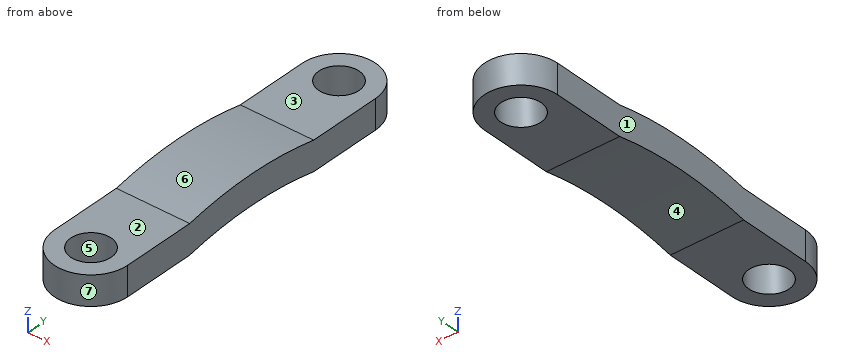
```python
from build123d import *

# Parameters (mm, degrees)
F1_DEPTH = 4
F2_D     = 5.5
F2_DEPTH = 7
F2_TIP   = 1.6523667023
F3_W     = 5
F3_H     = 4
F4_DEPTH = 5
F6_DEPTH = 4
F7_D     = 5.5
F7_DEPTH = 7
F7_TIP   = 1.6523667023


with BuildPart() as f1:
    # F0 (on Top) → F1 (new body)
    with BuildSketch(Plane.XY):
        with BuildLine():
            Line((-5, 5), (-5, 0))
            ThreePointArc((-5, 0), (0, -5), (5, 0))
            Line((5, 0), (5, 5))
            Line((5, 5), (-5, 5))
        make_face()
    extrude(amount=F1_DEPTH)

    # F2
    with Locations(Plane(origin=(0, 0, 0), x_dir=(1, 0, 0), z_dir=(0, 0, -1))):
        with Locations((0, 0)):
            Hole(F2_D / 2, depth=F2_DEPTH)
            with Locations((0, 0, -(F2_DEPTH + F2_TIP / 2))):  # 118° drill point
                Cone(0, F2_D / 2, F2_TIP, mode=Mode.SUBTRACT)

    # F3 (on Right) → F4 (join, symmetric)
    with BuildSketch(Plane.YZ):
        with Locations((7.5, 2)):
            Rectangle(F3_W, F3_H)
        with BuildLine():
            Line((10, 4), (10, 0))
            ThreePointArc((10, 0), (14.9745518997, 0.7570127946), (20, 1.0102051443))
            Line((20, 1.0102051443), (20, 5.0102051443))
            ThreePointArc((20, 5.0102051443), (14.9745518997, 4.7570127946), (10, 4))
        make_face()
        with BuildLine():
            Line((20, 5.0102051443), (20, 1.0102051443))
            ThreePointArc((20, 1.0102051443), (25.0254481003, 0.7570127946), (30, 0))
            Line((30, 0), (30, 4))
            ThreePointArc((30, 4), (25.0254481003, 4.7570127946), (20, 5.0102051443))
        make_face()
        with Locations((32.5, 2)):
            Rectangle(F3_W, F3_H)
    extrude(amount=F4_DEPTH, both=True)

    # F5 (on Top) → F6 (join)
    with BuildSketch(Plane.XY):
        with BuildLine():
            Line((5, 35), (5, 40))
            ThreePointArc((5, 40), (0, 45), (-5, 40))
            Line((-5, 40), (-5, 35))
            Line((-5, 35), (5, 35))
        make_face()
    extrude(amount=F6_DEPTH)

    # F7
    with Locations(Plane(origin=(0, 0, 0), x_dir=(1, 0, 0), z_dir=(0, 0, -1))):
        with Locations((0, -40)):
            Hole(F7_D / 2, depth=F7_DEPTH)
            with Locations((0, 0, -(F7_DEPTH + F7_TIP / 2))):  # 118° drill point
                Cone(0, F7_D / 2, F7_TIP, mode=Mode.SUBTRACT)


solid = f1.part
```
Model file for the job. Use its own axes, mm. Face numbers are marked on the shaded views. A direction names the side the tool comes from. Round coordinates to 2 decimals unless told otherwise and drop trailing zeros. Order: outer loops, then holes, each group sorted by start corner. A loop starts at its lowest first (then second) coordinate and runs counter-clockwise, first axis right, second up. Notation, with made-up numbers: (-39.75, 25) -> (-24.75, 25) arc R16 cw to (-24.75, 47) -> close; hole circle Ø6 at (69, 78.5). An arc over 180 degrees is marked (long way). Use one line per item in the form item = value.
Item 1: Cut at B-B, the plane x = 0. Write the cut outline in (y, z), and give its area (3 significant figures).
Returned:
outline = (-5, 0) -> (-2.75, 0) -> (-2.75, 4) -> (-5, 4) -> close; (2.75, 0) -> (10, 0) arc R50 cw to (30, 0) -> (37.25, 0) -> (37.25, 4) -> (30, 4) arc R50 ccw to (10, 4) -> (2.75, 4) -> close; (42.75, 0) -> (45, 0) -> (45, 4) -> (42.75, 4) -> close
area = 156 mm^2
Item 2: Cut at A-A, the plane z = 0.45. Write the cut outline in (x, y).
Returned:
outline = (-5, 0) arc R5 ccw to (5, 0) -> (5, 12.54) -> (-5, 12.54) -> close; (-5, 27.46) -> (5, 27.46) -> (5, 40) arc R5 ccw to (-5, 40) -> close; hole circle Ø5.5 at (0, 0); hole circle Ø5.5 at (0, 40)
Item 3: Pull direction Y, two halves, no side cores. Call the marked faces 4, 5, 6 and 7: released by +Y, released by -Y, zero draft, split by the parting line, or undercut.
Returned:
face_4 = undercut
face_5 = undercut
face_6 = split by the parting line
face_7 = released by -Y
Item 4: Flat gauge pins, fed straight in: pin 1 Ø3 at (x, y) = (-0.5, 6) entering from +Z; pin 2 Ø1.5 at (x, z) = (4, 2.5) entering from +Y; pin 3 Ø2 at (x, y) = (-1.5, 16) entering from -Z. Where does each tip first touch, or does it go through?
Returned:
pin_1 = 4
pin_2 = 43.8
pin_3 = 0.76
Item 5: Tool access for the marked faces 1, 2 and 3: list every direction of +Z, -Z, +X, -X, +Y, -Y with a clear straight run to the whole face (end or side of a thin tool).
Returned:
face_1 = +Z, -Z, -X, +Y, -Y
face_2 = +Z, +X, -X, -Y
face_3 = +Z, +X, -X, +Y
Item 6: Drill centre lines: line 1 (Y direction, x = 0, z = 1.7); line 2 (X direction, y = 40, z = 1.6); line 3 (Z direction, x = 2.5, y = 8). Where is each one in solid material? Low to high.
Returned:
line_1 = -5 to -2.75, 2.75 to 37.25, 42.75 to 45
line_2 = -5 to -2.75, 2.75 to 5
line_3 = 0 to 4
Item 7: Cut at D-D, the plane z = 3. Write the cut outline in (x, y), and give its area (3 significant figures).
Returned:
outline = (-5, 0) arc R5 ccw to (5, 0) -> (5, 40) arc R5 ccw to (-5, 40) -> close; hole circle Ø5.5 at (0, 0); hole circle Ø5.5 at (0, 40)
area = 431 mm^2
Item 8: Cut at C-C, the plane y = 1.5. Write the cut outline in (x, z), and give its area (3 significant figures).
Returned:
outline = (-5, 0) -> (-2.3, 0) -> (-2.3, 4) -> (-5, 4) -> close; (2.3, 0) -> (5, 0) -> (5, 4) -> (2.3, 4) -> close
area = 21.6 mm^2
